from build123d import *

# Parameters (mm, degrees)
SKETCH_1_W          = 25
SKETCH_1_H          = 21
EXTRUDE_1_DEPTH     = 3
CUT_EXTRUDE_1_REACH = 34.787
SKETCH_2_R          = 1.7


with BuildPart() as part:
    # 草图1 → 凸台-拉伸1 (new body)
    with BuildSketch(Plane.XY):
        with Locations((12.5, 10.5)):
            Rectangle(SKETCH_1_W, SKETCH_1_H)
    extrude(amount=EXTRUDE_1_DEPTH)

    # 草图2 → 切除-拉伸1 (cut, up to next)
    with BuildSketch(Plane.XY.offset(3), mode=Mode.PRIVATE) as cut_extrude_1_sk1:
        with Locations((20, 18)):
            Circle(SKETCH_2_R)
    cut_extrude_1_tool1 = extrude(cut_extrude_1_sk1.sketch, amount=-CUT_EXTRUDE_1_REACH, mode=Mode.PRIVATE) & part.part
    # 草图2 → 切除-拉伸1 (cut, up to next)
    with BuildSketch(Plane.XY.offset(3), mode=Mode.PRIVATE) as cut_extrude_1_sk2:
        with Locations((5, 18)):
            Circle(SKETCH_2_R)
    cut_extrude_1_tool2 = extrude(cut_extrude_1_sk2.sketch, amount=-CUT_EXTRUDE_1_REACH, mode=Mode.PRIVATE) & part.part
    # 草图2 → 切除-拉伸1 (cut, up to next)
    with BuildSketch(Plane.XY.offset(3), mode=Mode.PRIVATE) as cut_extrude_1_sk3:
        with Locations((5, 3)):
            Circle(SKETCH_2_R)
    cut_extrude_1_tool3 = extrude(cut_extrude_1_sk3.sketch, amount=-CUT_EXTRUDE_1_REACH, mode=Mode.PRIVATE) & part.part
    # 草图2 → 切除-拉伸1 (cut, up to next)
    with BuildSketch(Plane.XY.offset(3), mode=Mode.PRIVATE) as cut_extrude_1_sk4:
        with Locations((20, 3)):
            Circle(SKETCH_2_R)
    cut_extrude_1_tool4 = extrude(cut_extrude_1_sk4.sketch, amount=-CUT_EXTRUDE_1_REACH, mode=Mode.PRIVATE) & part.part
    add(cut_extrude_1_tool1.solids().sort_by_distance((20, 18, 3))[0], mode=Mode.SUBTRACT)
    add(cut_extrude_1_tool2.solids().sort_by_distance((5, 18, 3))[0], mode=Mode.SUBTRACT)
    add(cut_extrude_1_tool3.solids().sort_by_distance((5, 3, 3))[0], mode=Mode.SUBTRACT)
    add(cut_extrude_1_tool4.solids().sort_by_distance((20, 3, 3))[0], mode=Mode.SUBTRACT)


solid = part.part
Verification items for the finished model (mm, model axes). Give positions to 0.01 mm unless a question says otherwise; leave off trailing zeros. Write each loop counter-clockwise with the first axis right and the second up, starting at its lowest first coordinate (ties: lowest second). Pieces come first, ordered by that corner, then holes.
(1) Mould release check, pull along X, two halves, no side actions. Record for faces 1 (the face through (6.62, 3.51, 1.52)), 2 (the face through (12, 0, 1)), 3 (the face through (0, 10, 1)), 4 (the face through (25, 10, 1)): +X half, -X half, draft (parallel to the pull), parting line (faces both ways), or undercut.
(2) Cross-section at C-C (z = 0.4). Enter the section's corners in (x, y), plus the area to 3 significant figures.
(3) Material ranges on line 1 (Y direction, x = 5, z = 1.4); line 2 (X direction, y = 17.5, z = 1.7); line 3 (X direction, y = 16.5, z = 1), recorded low to high.
(4) Gauge pin test, flat end, axial feed: pin 1 (2 mm diameter, centred on x = 20, y = 3, fed in from +Z). Record the tip position at first contact, or that the pin passes through.
(5) Cross-section at B-B (x = 20). Enter the section's corners in (y, z).
(6) Cross-section at A-A (y = 3). Enter the section's corners in (x, z).
Worked out:
1. face 1: undercut
1. face 2: draft
1. face 3: -X half
1. face 4: +X half
2. outline: (0, 0) - (25, 0) - (25, 21) - (0, 21) - close; hole circle Ø3.4 at (5, 3); hole circle Ø3.4 at (5, 18); hole circle Ø3.4 at (20, 3); hole circle Ø3.4 at (20, 18)
2. area: 489 mm2
3. line 1: y = 0 to 1.3, 4.7 to 16.3, 19.7 to 21
3. line 2: x = 0 to 3.38, 6.62 to 18.38, 21.62 to 25
3. line 3: x = 0 to 4.2, 5.8 to 19.2, 20.8 to 25
4. pin 1: passes through
5. outline: (0, 0) - (1.3, 0) - (1.3, 3) - (0, 3) - close; (4.7, 0) - (16.3, 0) - (16.3, 3) - (4.7, 3) - close; (19.7, 0) - (21, 0) - (21, 3) - (19.7, 3) - close
6. outline: (0, 0) - (3.3, 0) - (3.3, 3) - (0, 3) - close; (6.7, 0) - (18.3, 0) - (18.3, 3) - (6.7, 3) - close; (21.7, 0) - (25, 0) - (25, 3) - (21.7, 3) - close
